from build123d import *

# Parameters (mm, degrees)
F0_W     = 20
F0_H     = 50
F1_DEPTH = 15
F2_W     = 10
F2_H     = 7
F2_H_2   = 33
F3_DEPTH = 20.001
F5_DEPTH = 15.001
F6_R     = 2
F7_DEPTH = 50.001
F8_R     = 1
F9_R     = 0.99999


# Not quite as in the source:
# - a fillet or chamfer is up to 0.001 mm smaller than in the source, because OpenCascade refuses the exact size


with BuildPart() as f1:
    # F0 (on Front) → F1 (new body)
    with BuildSketch(Plane.XZ):
        Rectangle(F0_W, F0_H)
    extrude(amount=F1_DEPTH)

    # F2 (on face) → F3 (cut, through all)
    with BuildSketch(Plane.YZ.offset(10)):
        with Locations((-10, 16.5)):
            Rectangle(F2_W, F2_H)
        with Locations((-10, -8.5)):
            Rectangle(F2_W, F2_H_2)
    extrude(amount=-F3_DEPTH, mode=Mode.SUBTRACT)

    # F4 (on face) → F5 (cut, through all)
    with BuildSketch(Plane(origin=(0, 0, 0), x_dir=(-1, 0, 0), z_dir=(0, 1, 0))):
        Polygon((0, -25), (-10, 0), (-10, -25), align=None)
        Polygon((10, 0), (0, -25), (10, -25), align=None)
    extrude(amount=-F5_DEPTH, mode=Mode.SUBTRACT)

    # F6 (on face) → F7 (cut, through all)
    with BuildSketch(Plane.XY.offset(25)):
        with Locations((0, -10)):
            Circle(F6_R)
    extrude(amount=-F7_DEPTH, mode=Mode.SUBTRACT)

    # F8
    f8_edges = [f1.edges().sort_by_distance(p)[0] for p in [
        (0, 0, 25),
        (10, -7.5, 25),
        (-10, -7.5, 25),
        (0, -15, 25),
        (10, 0, 12.5),
        (-10, 0, 12.5),
        (-10, -10, 8),
        (10, -10, 8),
        (0, -15, 8),
    ]]
    fillet(f8_edges, radius=F8_R)

    # F9 (radius 1 in the source; OpenCascade refuses exactly that, so slightly less here)
    f9_edges = [f1.edges().sort_by_distance(p)[0] for p in [
        (0, -15, 13),
        (0, -15, 20),
        (-10, -5, 4),
        (10, -5, 4),
    ]]
    fillet(f9_edges, radius=F9_R)


solid = f1.part
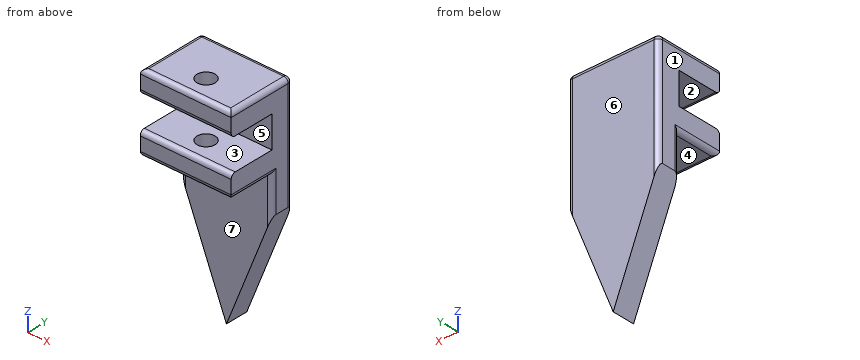
Here's how the part is built. I have some questions about the finished solid (model axes, mm). Face numbers are marked on the shaded views. A direction names the side the tool comes from. Give positions to 0.01 mm unless a question says otherwise; leave off trailing zeros. Loops run counter-clockwise (first coordinate to the right, second up) from the corner with the lowest first, then second, coordinate; pieces in that order, holes last. Notation, with made-up numbers: (8.5, -29) -> (36.5, -29) arc R24 cw to (36.5, 8) -> close; hole circle Ø8 at (18.5, 36.5). An arc over 180 degrees is marked (long way). Answer as a JSON object with one key per item and string values. Group by question number.
Item 1: Imagine slicing it at A-A on x = 8.5. Write out the boundary of the cut face in (y, z), then the cut area to 3 significant figures.
Item 2: I need wall thicknesses on L1, parallel to Y at x = 0, z = 10.2; L2, parallel to Z at x = 2, y = -7.5; L3, parallel to Y at x = 6.75, z = 18.5. Which ranges of each line are inside material? Lowest first, please.
Item 3: Imagine slicing it at B-B on y = -10. Write out the boundary of the cut face in (x, z).
Item 4: Imagine slicing it at D-D on y = -4.5. Write out the boundary of the cut face in (x, z).
Item 5: Imagine slicing it at C-C on z = 10. Write out the boundary of the cut face in (x, y), then the cut area to 3 significant figures.
Item 6: Will these pins go through, and if not, where does the flat tip stop? pin 1 (5 mm diameter, centred on x = 0, y = -10, fed in from -Z); pin 2 (2 mm diameter, centred on x = 1.5, z = 15.5, fed in from -Y); pin 3 (2 mm diameter, centred on x = 4, y = -1.5, fed in from -Z).
Item 7: On a 3-axis mill with a long thin cutter (end or side, diameter ignored), from which of +Z, -Z, +X, -X, +Y, -Y can I reach the whole of each face in a straight line? I mean the marked faces 5, 6 and 7. Say none if no direction works.
Item 8: Thinking about a two-plate mould opening in Z: for the marked faces 1, 2, 3 and 4, which applies, pulls with the +Z half, pulls with the -Z half, needs draft (parallel to the pull), parting line crosses it, or undercut?
Answer list:
{
 "1": {"outline": "(-15, 9) arc R1 ccw to (-14, 8) -> (-5, 8) -> (-5, -3.75) -> (0, -3.75) -> (0, 24) arc R1 ccw to (-1, 25) -> (-14, 25) arc R1 ccw to (-15, 24) -> (-15, 21) arc R1 ccw to (-14, 20) -> (-5, 20) -> (-5, 13) -> (-14, 13) arc R1 ccw to (-15, 12) -> close", "area": "243 mm2"},
 "2": {"L1": "y = -15 to -12, -8 to 0", "L2": "z = 8 to 13, 20 to 25", "L3": "y = -5 to 0"},
 "3": {"outline": "(-10, 9) arc R1 ccw to (-9, 8) -> (-2, 8) -> (-2, 13) -> (-10, 13) -> close; (-10, 20) -> (-2, 20) -> (-2, 25) -> (-9, 25) arc R1 ccw to (-10, 24) -> close; (2, 8) -> (9, 8) arc R1 ccw to (10, 9) -> (10, 13) -> (2, 13) -> close; (2, 20) -> (10, 20) -> (10, 24) arc R1 ccw to (9, 25) -> (2, 25) -> close"},
 "4": {"outline": "(-10, 9) arc R1 ccw to (-9.87, 8.5) -> (-9.87, -0.33) -> (0, -25) -> (9.87, -0.33) -> (9.87, 8.5) arc R1 ccw to (10, 9) -> (10, 24) arc R1 ccw to (9, 25) -> (-9, 25) arc R1 ccw to (-10, 24) -> close"},
 "5": {"outline": "(-10, -15) -> (10, -15) -> (10, -1) arc R1 ccw to (9, 0) -> (-9, 0) arc R1 ccw to (-10, -1) -> close; hole circle Ø4 at (0, -10)", "area": "287 mm2"},
 "6": {"pin 1": "stops at z = 8", "pin 2": "stops at y = -5", "pin 3": "stops at z = -17.5"},
 "7": {"face 5": "+X, -X, -Y", "face 6": "+Z, -Z, +X, -X, +Y", "face 7": "-Z, +X, -X, -Y"},
 "8": {"face 1": "needs draft", "face 2": "undercut", "face 3": "undercut", "face 4": "pulls with the -Z half"}
}
